```python
from build123d import *

# Parameters (mm, degrees)
SKETCH_1_R          = 3
EXTRUDE_1_DEPTH     = 2
SKETCH_2_R          = 4
SKETCH_2_W          = 27.67766953
SKETCH_2_H          = 2
EXTRUDE_2_DEPTH     = 2
EXTRUDE_START       = 2
SKETCH_3_W          = 55.35533906
SKETCH_3_H          = 26
SKETCH_3_R          = 4
EXTRUDE_3_DEPTH     = 2
SKETCH_4_W          = 55.35533906
SKETCH_4_H          = 24
CUT_EXTRUDE_1_DEPTH = 2
FILLET_1_R          = 2
SKETCH_5_W          = 55.35533906
SKETCH_5_H          = 2
EXTRUDE_4_DEPTH     = 22
SKETCH_6_R          = 1.3
CUT_EXTRUDE_2_DEPTH = 22
FILLET_2_R          = 2
FILLET_3_R          = 2
FILLET_4_R          = 2


with BuildPart() as part:
    # 草图1 → 凸台-拉伸1 (new body)
    with BuildSketch(Plane(origin=(0, 0, 0), x_dir=(1, 0, 0), z_dir=(0, 1, 0))):
        Polygon((-17.67766953, 9.67766953), (-27.67766953, 9.67766953), (-27.67766953, 25.67766953), (17.67766953, 25.67766953), (27.67766953, 25.67766953), (27.67766953, 9.67766953), align=None)
        with Locations(Location((-17.67766953, 17.67766953, 0), (0, 0, 270))):
            Circle(SKETCH_1_R, mode=Mode.SUBTRACT)
        with Locations(Location((17.67766953, 17.67766953, 0), (0, 0, 270))):
            Circle(SKETCH_1_R, mode=Mode.SUBTRACT)
    extrude(amount=EXTRUDE_1_DEPTH)

    # 草图2 → 凸台-拉伸2 (add)
    # profile 1 of 3: a face of its own
    with BuildSketch(Plane.XY.offset(-9.67766953)):
        Polygon((-27.67766953, 26), (-27.67766953, 2), (0, 2), (27.67766953, 2), (27.67766953, 26), align=None)
        with Locations((-9, 14)):
            Circle(SKETCH_2_R, mode=Mode.SUBTRACT)
        with Locations((9, 14)):
            Circle(SKETCH_2_R, mode=Mode.SUBTRACT)
    # profile 2 of 3: a face of its own
    with BuildSketch(Plane.XY.offset(-9.67766953)):
        with Locations((-13.838834765, 1)):
            Rectangle(SKETCH_2_W, SKETCH_2_H)
    # profile 3 of 3: a face of its own
    with BuildSketch(Plane.XY.offset(-9.67766953)):
        with Locations((13.838834765, 1)):
            Rectangle(SKETCH_2_W, SKETCH_2_H)
    extrude(amount=-EXTRUDE_2_DEPTH)

    # 草图3 → 凸台-拉伸3 (add)
    with BuildSketch(Plane.XY.offset(-9.67766953).offset(EXTRUDE_START)):
        with Locations((0, 13)):
            Rectangle(SKETCH_3_W, SKETCH_3_H)
        with Locations((-9, 14)):
            Circle(SKETCH_3_R, mode=Mode.SUBTRACT)
        with Locations((9, 14)):
            Circle(SKETCH_3_R, mode=Mode.SUBTRACT)
    extrude(amount=-EXTRUDE_3_DEPTH)

    # 草图4 → 切除-拉伸1 (cut)
    with BuildSketch(Plane.XY.offset(-9.67766953)):
        with Locations((0, 14)):
            Rectangle(SKETCH_4_W, SKETCH_4_H)
    extrude(amount=-CUT_EXTRUDE_1_DEPTH, mode=Mode.SUBTRACT)

    # 圆角1
    fillet_1_edges = [part.edges().sort_by_distance(p)[0] for p in [
        (0, 0, -7.67766953),
    ]]
    fillet(fillet_1_edges, radius=FILLET_1_R)

    # 草图5 → 凸台-拉伸4 (add)
    with BuildSketch(Plane(origin=(0, 0, -9.67766953), x_dir=(-1, 0, 0), z_dir=(0, 0, -1))):
        with Locations((0, 27)):
            Rectangle(SKETCH_5_W, SKETCH_5_H)
    extrude(amount=-EXTRUDE_4_DEPTH)

    # 草图6 → 切除-拉伸2 (cut)
    with BuildSketch(Plane(origin=(0, 28, 0), x_dir=(1, 0, 0), z_dir=(0, 1, 0))):
        with Locations(Location((25, -8, 0), (0, 0, 270))):
            Circle(SKETCH_6_R)
        with Locations(Location((25, 4, 0), (0, 0, 270))):
            Circle(SKETCH_6_R)
        with Locations(Location((-25, 4, 0), (0, 0, 90))):
            Circle(SKETCH_6_R)
        with Locations(Location((-25, -8, 0), (0, 0, 90))):
            Circle(SKETCH_6_R)
    extrude(amount=-CUT_EXTRUDE_2_DEPTH, mode=Mode.SUBTRACT)

    # 圆角2
    fillet_2_edges = [part.edges().sort_by_distance(p)[0] for p in [
        (0, 28, -9.67766953),
    ]]
    fillet(fillet_2_edges, radius=FILLET_2_R)

    # 圆角3
    fillet_3_edges = [part.edges().sort_by_distance(p)[0] for p in [
        (0, 26, -7.67766953),
    ]]
    fillet(fillet_3_edges, radius=FILLET_3_R)

    # 圆角4
    fillet_4_edges = [part.edges().sort_by_distance(p)[0] for p in [
        (0, 2, -9.67766953),
    ]]
    fillet(fillet_4_edges, radius=FILLET_4_R)


solid = part.part
```
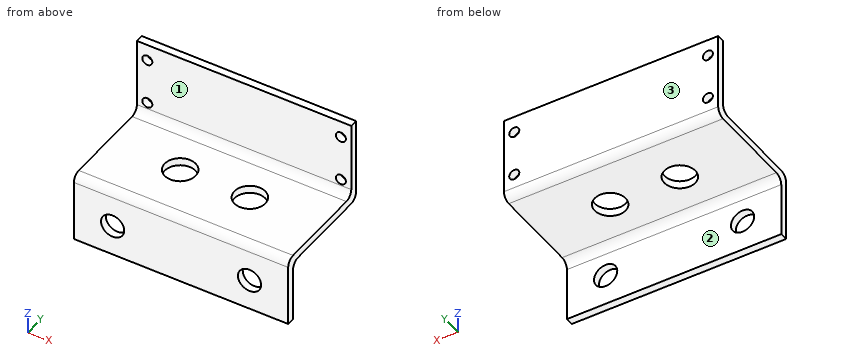
Can you work these out from the model? Positions are in its coordinate system, mm. Face numbers are marked on the shaded views. A direction names the side the tool comes from. Give positions to 0.01 mm unless a question says otherwise; leave off trailing zeros. Loops run counter-clockwise (first coordinate to the right, second up) from the corner with the lowest first, then second, coordinate; pieces in that order, holes last. Notation, with made-up numbers: M 13.25,76 L 70.25,76 A34 ccw 70.25,114 Z; hole C 38,67 d9. An arc over 180 degrees is marked long. Use CSV: the item, a comma, the result in double quotes. Start each with the question number.
1. For P1, Ø9, axis at x = -9, y = 14, coming from the -Z side; P2, Ø3.5, axis at x = -25, z = -4, coming from the +Y side; P3, Ø7, axis at x = -17.68, z = -17.68, coming from the +Y side; P4, Ø3, axis at x = -25, z = 8, coming from the -Y side, each with a flat end and sliding along its axis, tell me the tip position at first contact or that it passes through.
2. If I drill on L1, parallel to X at y = 26.6, z = -4; L2, parallel to Z at x = -25, y = 27.25; L3, parallel to Z at x = -25, y = 26.9, over which ranges is the centre line in solid material (lowest first)?
3. On a 3-axis mill with a long thin cutter (end or side, diameter ignored), from which of +Z, -Z, +X, -X, +Y, -Y can I reach the whole of each face in a straight line? I mean the marked faces 1, 2 and 3. Say none if no direction works.
4. Imagine slicing it at C-C, the plane x = -9. Write out the boundary of the cut face in (y, z), plus the area to 3 significant figures.
5. Imagine slicing it at A-A, the plane z = 8. Write out the boundary of the cut face in (x, y).
6. Imagine slicing it at B-B, the plane y = 14. Write out the boundary of the cut face in (x, z).
7. Imagine slicing it at D-D, the plane x = -25. Write out the boundary of the cut face in (y, z), plus the area to 3 significant figures.
Response values:
1,P1,"z = -9.68"
1,P2,"y = 28"
1,P3,"y = 2"
1,P4,"y = 26"
2,L1,"-27.68 to -26.3, -23.7 to 23.7, 26.3 to 27.68"
2,L2,"-9.24 to -5.3, -2.7 to 6.7, 9.3 to 12.32"
2,L3,"-9.46 to -5.3, -2.7 to 6.7, 9.3 to 12.32"
3,face 1,"+Z, +X, -X, -Y"
3,face 2,"-Z, +X, -X, +Y"
3,face 3,"+Z, -Z, +X, -X, +Y"
4,outline,"M 0,-25.68 L 2,-25.68 L 2,-11.68 A2 cw 4,-9.68 L 10,-9.68 L 10,-7.68 L 2,-7.68 A2 ccw 0,-9.68 Z; M 18,-9.68 L 26,-9.68 A2 ccw 28,-7.68 L 28,12.32 L 26,12.32 L 26,-5.68 A2 cw 24,-7.68 L 18,-7.68 Z"
4,area,"112 mm^2"
5,outline,"M -27.68,26 L -26.3,26 L -26.3,28 L -27.68,28 Z; M -23.7,26 L 23.7,26 L 23.7,28 L -23.7,28 Z; M 26.3,26 L 27.68,26 L 27.68,28 L 26.3,28 Z"
6,outline,"M -27.68,-9.68 L -13,-9.68 L -13,-7.68 L -27.68,-7.68 Z; M -5,-9.68 L 5,-9.68 L 5,-7.68 L -5,-7.68 Z; M 13,-9.68 L 27.68,-9.68 L 27.68,-7.68 L 13,-7.68 Z"
7,outline,"M 0,-25.68 L 2,-25.68 L 2,-11.68 A2 cw 4,-9.68 L 26,-9.68 A2 ccw 28,-7.68 L 28,-5.3 L 26,-5.3 L 26,-5.68 A2 cw 24,-7.68 L 2,-7.68 A2 ccw 0,-9.68 Z; M 26,-2.7 L 28,-2.7 L 28,6.7 L 26,6.7 Z; M 26,9.3 L 28,9.3 L 28,12.32 L 26,12.32 Z"
7,area,"118 mm^2"
